from build123d import *

# Parameters (mm, degrees)
F0_W     = 121.257108
F0_H     = 111.767154
F1_DEPTH = 35.306
F2_R     = 24.891724
F3_DEPTH = 31.75
F5_DEPTH = 152.654


with BuildPart() as f1:
    # F0 (on Top) → F1 (new body)
    with BuildSketch(Plane.XY):
        with Locations((4.806647, -6.510528)):
            Rectangle(F0_W, F0_H)
    extrude(amount=F1_DEPTH)

    # F2 (on face) → F3 (join)
    with BuildSketch(Plane.XY.offset(35.306)):
        Circle(F2_R)
    extrude(amount=F3_DEPTH)

    # F4 (on face) → F5 (cut)
    with BuildSketch(Plane.XZ.offset(62.394105)):
        Polygon((-27.139649, 79.367436), (-25.687542, 67.387573), (32.396633, 50.325349), (32.396633, 79.367436), align=None)
    extrude(amount=-F5_DEPTH, mode=Mode.SUBTRACT)


solid = f1.part
The model under review builds one solid part; all positions refer to its coordinate system, in mm. A direction names the side the tool comes from. Give positions to 0.01 mm unless a question says otherwise; leave off trailing zeros. Write each loop counter-clockwise with the first axis right and the second up, starting at its lowest first coordinate (ties: lowest second). Pieces come first, ordered by that corner, then holes.
1. Add section A-A, the plane y = 0. Write out the cut boundary in (x, z), plus the area to 3 significant figures.
2. For P1, Ø4, axis at x = 14.5, z = 45.5, coming from the -Y side; P2, Ø4, axis at x = 4, y = -44.5, coming from the +Z side; P3, Ø3, axis at y = -6.5, z = 46.5, coming from the -X side, all flat-tipped, find the tip position at first contact; note any pin that passes through.
3. Add section C-C, the plane z = 39.5. Write out the cut boundary in (x, y).
4. Add section B-B, the plane x = 0. Write out the cut boundary in (y, z), plus the area to 3 significant figures.
5. Add section D-D, the plane x = -44. Write out the cut boundary in (y, z), plus the area to 3 significant figures.
6. Tool access review of faces 1 (the flat face through (17.4, -18.1, 35.306)), 2 (the flat face through (-0.2, -0.3, 59.9)): name each direction out of +Z, -Z, +X, -X, +Y, -Y from which nothing blocks a thin tool from reaching the whole face with its end or side.
7. Wall thickness on L1, parallel to Z at x = -37, y = -30; L2, parallel to Y at x = 0.5, z = 50; L3, parallel to Z at x = 4.5, y = 23: over which ranges is each line inside the solid? List them lowest first.
Worked answers:
1. outline: (-55.82, 0) - (65.44, 0) - (65.44, 35.31) - (24.89, 35.31) - (24.89, 52.53) - (-24.56, 67.06) - (-24.89, 67.06) - (-24.89, 35.31) - (-55.82, 35.31) - close
1. area: 5,500 mm2
2. P1: stops at y = -21.53
2. P2: stops at z = 35.31
2. P3: stops at x = -24.38
3. outline: circle Ø49.78 at (0, 0)
4. outline: (-62.39, 0) - (49.37, 0) - (49.37, 35.31) - (24.89, 35.31) - (24.89, 59.84) - (-24.89, 59.84) - (-24.89, 35.31) - (-62.39, 35.31) - close
4. area: 5,170 mm2
5. outline: (-62.39, 0) - (49.37, 0) - (49.37, 35.31) - (-62.39, 35.31) - close
5. area: 3,950 mm2
6. face 1: +Z
6. face 2: +Z, +X, +Y, -Y
7. L1: z = 0 to 35.31
7. L2: y = -24.89 to 24.89
7. L3: z = 0 to 58.52
